Design review of the part built by this model. Coordinates are the model's own, in mm. A direction names the side the tool comes from. Round coordinates to 2 decimals unless told otherwise and drop trailing zeros. Loops run counter-clockwise (first coordinate to the right, second up) from the corner with the lowest first, then second, coordinate; pieces in that order, holes last. Notation, with made-up numbers: (56, 19.25) - (109, 19.25) arc R22 cw to (109, 53.25) - close; hole circle Ø7 at (-12.75, 48.5). An arc over 180 degrees is marked (long way). Return JSON: item names as keys, results as strings. Group by question number.
(1) We need section A-A, the plane z = -4.73. Write out the cut boundary in (x, y) (3 decimals).
(2) We need section C-C, the plane y = 4. Write out the cut boundary in (x, z).
(3) Clearance check with flat-ended pins moving along their axes: pin 1 (6.5 mm diameter, centred on x = 13, z = -8, fed in from +Y); pin 2 (1 mm diameter, centred on x = 14, z = -7.27, fed in from +Y); pin 3 (2 mm diameter, centred on x = 6, z = -4.73, fed in from +Y). State where each tip first meets the part, or that it passes through.
(4) We need section D-D, the plane z = -9.5. Write out the cut boundary in (x, y), and give its area (3 significant figures).
(5) Wall thickness on L1, parallel to Z at x = 14, y = 0.9 (3 decimals); L2, parallel to X at y = 9.25, z = -7; L3, parallel to Z at x = 11.75, y = 6: over which ranges is each line inside the solid? List them lowest first. Write a range as [from, to].
(6) The part is to be moulded in two halves that separate along Z. For faces 3 (the flat face through (0.5, 6, -6)), 4 (the flat face through (10, 6, -11.5)), 5 (the cylindrical face through (14.336, 1.24, -4.203)), say which applies: pulls with the +Z half, pulls with the -Z half, needs draft (parallel to the pull), parting line crosses it, or undercut.
(7) For faces 1 (the flat face through (10, 6, -10)), 2 (the flat face through (10, 11, -1)), list the 3-axis set-ups (+Z, -Z, +X, -X, +Y, -Y) from which the entire face can be reached by the end or side of a thin tool; tool diameter is ignored.
(8) We need section B-B, the plane x = 14. Write out the cut boundary in (y, z) (3 decimals), and give its area (4 significant figures).
from build123d import *

# Parameters (mm, degrees)
SKETCH1_W           = 20
SKETCH1_H           = 12
BOSS_EXTRUDE1_DEPTH = 11
SHELL1_T            = -2
SKETCH3_R           = 0.625
CUT_EXTRUDE1_DEPTH  = 10
LPATTERN1_COUNT     = 2
LPATTERN1_PITCH     = 8
SKETCH5_W           = 20
SKETCH5_H           = 12
SKETCH5_W_2         = 19
SKETCH5_H_2         = 11
CUT_EXTRUDE2_DEPTH  = 12
SKETCH6_W           = 19
SKETCH6_H           = 11
CUT_EXTRUDE3_DEPTH  = 0.5


with BuildPart() as part:
    # Sketch1 → Boss-Extrude1 (new body)
    with BuildSketch(Plane(origin=(0, 0, 0), x_dir=(1, 0, 0), z_dir=(0, 1, 0))):
        with Locations((10, 6)):
            Rectangle(SKETCH1_W, SKETCH1_H)
    extrude(amount=BOSS_EXTRUDE1_DEPTH)

    # Shell1
    shell1_openings = [part.faces().sort_by_distance(p)[0] for p in [
        (10, 11, -6),
    ]]
    offset(amount=SHELL1_T, openings=shell1_openings, kind=Kind.INTERSECTION)

    # Sketch3 → Cut-Extrude1 (cut)
    with BuildSketch(Plane.XZ):
        with Locations((6, -4.73)):
            Circle(SKETCH3_R)
        with Locations((6, -7.27)):
            Circle(SKETCH3_R)
    cut_extrude1 = extrude(amount=-CUT_EXTRUDE1_DEPTH, mode=Mode.SUBTRACT)

    # LPattern1: Cut-Extrude1 ×2
    with Locations(*[(i * LPATTERN1_PITCH, 0, 0) for i in range(1, LPATTERN1_COUNT)]):
        add(cut_extrude1, mode=Mode.SUBTRACT)

    # Sketch5 → Cut-Extrude2 (cut, through all)
    with BuildSketch(Plane(origin=(0, 11, 0), x_dir=(1, 0, 0), z_dir=(0, 1, 0))):
        with Locations((10, 6)):
            Rectangle(SKETCH5_W, SKETCH5_H)
        with Locations((10, 6)):
            Rectangle(SKETCH5_W_2, SKETCH5_H_2, mode=Mode.SUBTRACT)
    extrude(amount=-CUT_EXTRUDE2_DEPTH, mode=Mode.SUBTRACT)

    # Sketch6 → Cut-Extrude3 (cut)
    with BuildSketch(Plane.XZ):
        with Locations((10, -6)):
            Rectangle(SKETCH6_W, SKETCH6_H)
    extrude(amount=-CUT_EXTRUDE3_DEPTH, mode=Mode.SUBTRACT)


solid = part.part
Solutions:
{
 "1": {"outline": "(0.5, 0.5) - (5.375, 0.5) - (5.375, 2) - (2, 2) - (2, 11) - (0.5, 11) - close; (6.625, 0.5) - (13.375, 0.5) - (13.375, 2) - (6.625, 2) - close; (14.625, 0.5) - (19.5, 0.5) - (19.5, 11) - (18, 11) - (18, 2) - (14.625, 2) - close"},
 "2": {"outline": "(0.5, -11.5) - (19.5, -11.5) - (19.5, -0.5) - (0.5, -0.5) - close; hole (2, -10) - (18, -10) - (18, -2) - (2, -2) - close"},
 "3": {"pin 1": "y = 11", "pin 2": "through", "pin 3": "y = 2"},
 "4": {"outline": "(0.5, 0.5) - (19.5, 0.5) - (19.5, 11) - (18, 11) - (18, 2) - (2, 2) - (2, 11) - (0.5, 11) - close", "area": "55.5 mm^2"},
 "5": {"L1": "[-11.5, -7.895], [-6.645, -5.355], [-4.105, -0.5]", "L2": "[0.5, 2], [18, 19.5]", "L3": "[-11.5, -10], [-2, -0.5]"},
 "6": {"face 3": "needs draft", "face 4": "pulls with the -Z half", "face 5": "undercut"},
 "7": {"face 1": "+Y", "face 2": "+Z, -Z, +X, -X, +Y"},
 "8": {"outline": "(0.5, -11.5) - (11, -11.5) - (11, -10) - (2, -10) - (2, -7.895) - (0.5, -7.895) - close; (0.5, -6.645) - (2, -6.645) - (2, -5.355) - (0.5, -5.355) - close; (0.5, -4.105) - (2, -4.105) - (2, -2) - (11, -2) - (11, -0.5) - (0.5, -0.5) - close", "area": "39.75 mm^2"}
}
